```python
from build123d import *

# Parameters (mm, degrees)
CROQUIS1_W              = 34
CROQUIS1_H              = 40
CROQUIS1_R              = 4.75
SALIENTE_EXTRUIR1_DEPTH = 16.5
CROQUIS2_R              = 8.25
CORTAR_EXTRUIR1_DEPTH   = 4.6
CROQUIS3_R              = 1.325
CORTAR_EXTRUIR2_DEPTH   = 5.6
CORTAR_EXTRUIR3_REACH   = 44.758
CROQUIS4_R              = 1.6
CROQUIS5_R              = 3.25
CORTAR_EXTRUIR4_DEPTH   = 28.6
REDONDEO1_R             = 5


with BuildPart() as part:
    # Croquis1 → Saliente-Extruir1 (new body)
    with BuildSketch(Plane.XY):
        Rectangle(CROQUIS1_W, CROQUIS1_H)
        with Locations((4, 0)):
            Circle(CROQUIS1_R, mode=Mode.SUBTRACT)
    extrude(amount=SALIENTE_EXTRUIR1_DEPTH)

    # Croquis2 → Cortar-Extruir1 (cut)
    with BuildSketch(Plane.XY.offset(16.5)):
        with Locations((4, 0)):
            Circle(CROQUIS2_R)
    extrude(amount=-CORTAR_EXTRUIR1_DEPTH, mode=Mode.SUBTRACT)

    # Croquis3 → Cortar-Extruir2 (cut)
    with BuildSketch(Plane(origin=(17, 0, 0), x_dir=(0, 0, -1), z_dir=(1, 0, 0))):
        with Locations(Location((-14.25, 0, 0), (0, 0, 90))):
            Circle(CROQUIS3_R)
    extrude(amount=-CORTAR_EXTRUIR2_DEPTH, mode=Mode.SUBTRACT)

    # Croquis4 → Cortar-Extruir3 (cut, up to next)
    with BuildSketch(Plane(origin=(17, 0, 0), x_dir=(0, 0, -1), z_dir=(1, 0, 0)), mode=Mode.PRIVATE) as cortar_extruir3_sk1:
        with Locations(Location((-8.25, -10, 0), (0, 0, 90))):
            Circle(CROQUIS4_R)
    cortar_extruir3_tool1 = extrude(cortar_extruir3_sk1.sketch, amount=-CORTAR_EXTRUIR3_REACH, mode=Mode.PRIVATE) & part.part
    # Croquis4 → Cortar-Extruir3 (cut, up to next)
    with BuildSketch(Plane(origin=(17, 0, 0), x_dir=(0, 0, -1), z_dir=(1, 0, 0)), mode=Mode.PRIVATE) as cortar_extruir3_sk2:
        with Locations(Location((-8.25, 10, 0), (0, 0, 90))):
            Circle(CROQUIS4_R)
    cortar_extruir3_tool2 = extrude(cortar_extruir3_sk2.sketch, amount=-CORTAR_EXTRUIR3_REACH, mode=Mode.PRIVATE) & part.part
    add(cortar_extruir3_tool1.solids().sort_by_distance((17, -10, 8.25))[0], mode=Mode.SUBTRACT)
    add(cortar_extruir3_tool2.solids().sort_by_distance((17, 10, 8.25))[0], mode=Mode.SUBTRACT)

    # Croquis5 → Cortar-Extruir4 (cut)
    with BuildSketch(Plane(origin=(17, 0, 0), x_dir=(0, 0, -1), z_dir=(1, 0, 0))):
        with Locations(Location((-8.25, -10, 0), (0, 0, 90))):
            Circle(CROQUIS5_R)
        with Locations(Location((-8.25, 10, 0), (0, 0, 90))):
            Circle(CROQUIS5_R)
    extrude(amount=-CORTAR_EXTRUIR4_DEPTH, mode=Mode.SUBTRACT)

    # Redondeo1
    redondeo1_edges = [part.edges().sort_by_distance(p)[0] for p in [
        (17, 20, 8.25),
        (17, -20, 8.25),
    ]]
    fillet(redondeo1_edges, radius=REDONDEO1_R)


solid = part.part
```
Geometry check sheet. Reference: the model listing, model coordinates, mm. A direction names the side the tool comes from. Give positions to 0.01 mm unless a question says otherwise; leave off trailing zeros. Loops run counter-clockwise (first coordinate to the right, second up) from the corner with the lowest first, then second, coordinate; pieces in that order, holes last. Notation, with made-up numbers: M -9,66 L 42,66 A13 ccw 42,80 Z; hole C 25.5,50 d7. An arc over 180 degrees is marked long. Answer as CSV lines item,"result".
Item 1: Depth check by flat-ended pin: P1, Ø12.5, axis at x = 4, y = 0, coming from the +Z side; P2, Ø4, axis at y = -10, z = 8.25, coming from the +X side. Enter the tip coordinate at first touch or a pass-through.
Values:
P1,"stops at z = 11.9"
P2,"stops at x = -11.6"
Item 2: Cross-section at D-D on x = -8.5. Record the cut outline in (y, z).
Values:
outline,"M -20,0 L 20,0 L 20,16.5 L -20,16.5 Z; hole C -10,8.25 d6.5; hole C 10,8.25 d6.5"
Item 3: Cross-section at B-B on y = -10. Record the cut outline in (x, z).
Values:
outline,"M -17,0 L 17,0 L 17,5 L -11.6,5 L -11.6,6.65 L -17,6.65 Z; M -17,9.85 L -11.6,9.85 L -11.6,11.5 L 17,11.5 L 17,16.5 L -17,16.5 Z"
Item 4: Release check for a two-part mould opening along Z. For faces 4 (the flat face through (17, 0, 8)), 5 (the flat face through (-4, 0, 0)), 6 (the cylindrical face through (-14.3, 8.4, 8.3)), 7 (the cylindrical face through (-14.3, -11.6, 8.3)) record: pulls with the +Z half, pulls with the -Z half, needs draft (parallel to the pull), parting line crosses it, or undercut.
Values:
face 4,"needs draft"
face 5,"pulls with the -Z half"
face 6,"undercut"
face 7,"undercut"
Item 5: Material ranges on line 1 (Y direction, x = 4, z = 13.4); line 2 (X direction, y = 0, z = 3); line 3 (Z direction, x = 6, y = 10), recorded low to high.
Values:
line 1,"y = -20 to -8.25, 8.25 to 20"
line 2,"x = -17 to -0.75, 8.75 to 17"
line 3,"z = 0 to 5, 11.5 to 16.5"
Item 6: Cross-section at C-C on x = 4. Record the cut outline in (y, z), and give its area (3 significant figures).
Values:
outline,"M -20,0 L -4.75,0 L -4.75,11.9 L -8.25,11.9 L -8.25,16.5 L -20,16.5 Z; M 4.75,0 L 20,0 L 20,16.5 L 8.25,16.5 L 8.25,11.9 L 4.75,11.9 Z; hole C -10,8.25 d6.5; hole C 10,8.25 d6.5"
area,"405 mm²"
Item 7: Cross-section at A-A on z = 8.25. Record the cut outline in (x, y), and give its area (3 significant figures).
Values:
outline,"M -17,-20 L 12,-20 A5 ccw 17,-15 L 17,-13.25 L -11.6,-13.25 L -11.6,-11.6 L -17,-11.6 Z; M -17,-8.4 L -11.6,-8.4 L -11.6,-6.75 L 17,-6.75 L 17,6.75 L -11.6,6.75 L -11.6,8.4 L -17,8.4 Z; M -17,11.6 L -11.6,11.6 L -11.6,13.25 L 17,13.25 L 17,15 A5 ccw 12,20 L -17,20 Z; hole C 4,0 d9.5"
area,"872 mm²"
Item 8: Access from +Z, -Z, +X, -X, +Y, -Y to the whole of each face (thin tool, end or side, straight path). Record for faces 1 (the cylindrical face through (-2.081, 5.576, 14.232)), 2 (the cylindrical face through (2.9, -12.395, 10.447)), 3 (the flat face through (-4, 5, 16.5)).
Values:
face 1,"+Z"
face 2,"+X"
face 3,"+Z, +X, -X, +Y, -Y"
